Model file for the job. Use its own axes, mm. Give positions to 0.01 mm unless a question says otherwise; leave off trailing zeros. Write each loop counter-clockwise with the first axis right and the second up, starting at its lowest first coordinate (ties: lowest second). Pieces come first, ordered by that corner, then holes. Notation, with made-up numbers: (12, -19.5) - (37, -19.5) arc R25 cw to (37, -5.5) - close; hole circle Ø3 at (72, -39.5). An arc over 180 degrees is marked (long way). Use CSV: the item, a comma, the result in double quotes.
from build123d import *

# Parameters (mm, degrees)
SKETCH1_W           = 560
SKETCH1_H           = 25
BOSS_EXTRUDE1_DEPTH = 16
FILLET1_R           = 8


with BuildPart() as part:
    # Sketch1 → Boss-Extrude1 (new body)
    with BuildSketch(Plane.XY):
        with Locations((0, 12.5)):
            Rectangle(SKETCH1_W, SKETCH1_H)
    extrude(amount=BOSS_EXTRUDE1_DEPTH)

    # Fillet1
    fillet1_edges = [part.edges().sort_by_distance(p)[0] for p in [
        (0, 25, 16),
    ]]
    fillet(fillet1_edges, radius=FILLET1_R)


solid = part.part
(1) Pull direction Z, two halves, no side cores. Call faces 1 (the face through (-4, 13, 0)), 2 (the face through (280, 12, 8)), 3 (the face through (-4, 9, 16)): released by +Z, released by -Z, zero draft, split by the parting line, or undercut.
Checked values:
face 1,"released by -Z"
face 2,"zero draft"
face 3,"released by +Z"
(2) Saw through at A-A, the plane x = -9. List the corners of the cut face in (y, z).
Checked values:
outline,"(0, 0) - (25, 0) - (25, 8) arc R8 ccw to (17, 16) - (0, 16) - close"
(3) Saw through at B-B, the plane z = 12.25. List the corners of the cut face in (x, y).
Checked values:
outline,"(-280, 0) - (280, 0) - (280, 23.78) - (-280, 23.78) - close"
(4) Wall check: probe 1 along Z at (x, y) = (-179.5, 17.5); probe 2 along Y at (x, z) = (256, 8.5); probe 3 along Y at (x, z) = (20, 9.5). Give the ranges that are in metal, low to high. Write a range as [from, to].
Checked values:
probe 1,"z = [0, 15.98]"
probe 2,"y = [0, 24.98]"
probe 3,"y = [0, 24.86]"
